```python
from build123d import *

# Parameters (mm, degrees)
BOSS_EXTRUDE1_DEPTH = 2
BOSS_EXTRUDE2_START = 10
SKETCH3_R           = 5
SKETCH3_R_2         = 3
BOSS_EXTRUDE2_DEPTH = 10
SKETCH4_R           = 5
SKETCH4_R_2         = 3
BOSS_EXTRUDE3_DEPTH = 10


with BuildPart() as part:
    # Sketch2 → Boss-Extrude1 (new, symmetric)
    with BuildSketch(Plane.XY):
        with BuildLine():
            Line((-17.054545455, 5), (7.945454545, 5))
            ThreePointArc((7.945454545, 5), (12.945454545, 0), (7.945454545, -5))
            Line((7.945454545, -5), (-17.054545455, -5))
            ThreePointArc((-17.054545455, -5), (-22.054545455, 0), (-17.054545455, 5))
        make_face()
    extrude(amount=BOSS_EXTRUDE1_DEPTH, both=True)

    # Sketch3 → Boss-Extrude2 (add)
    with BuildSketch(Plane.XY.offset(2).offset(BOSS_EXTRUDE2_START)):
        with Locations(Location((-17.054545455, 0, 0), (0, 0, 270))):
            Circle(SKETCH3_R)
        with Locations((-17.054545455, 0)):
            Circle(SKETCH3_R_2, mode=Mode.SUBTRACT)
    extrude(amount=-BOSS_EXTRUDE2_DEPTH)

    # Sketch4 → Boss-Extrude3 (add)
    with BuildSketch(Plane(origin=(0, 0, -2), x_dir=(-1, 0, 0), z_dir=(0, 0, -1))):
        with Locations((-7.945454545, 0)):
            Circle(SKETCH4_R)
        with Locations((-7.945454545, 0)):
            Circle(SKETCH4_R_2, mode=Mode.SUBTRACT)
    extrude(amount=BOSS_EXTRUDE3_DEPTH)


solid = part.part
```
Can you work these out from the model? Positions are in its coordinate system, mm. A direction names the side the tool comes from. Coordinates: 2 decimals unless noted, no trailing zeros. Write each loop counter-clockwise with the first axis right and the second up, starting at its lowest first coordinate (ties: lowest second). Pieces come first, ordered by that corner, then holes. Notation, with made-up numbers: M -11.75,-6 L 7.25,-6 A23 ccw 7.25,14 Z; hole C 54,-37.75 d8. An arc over 180 degrees is marked long. Write item = value, one per line. Start each with the question number.
Q1. On a 3-axis mill with a long thin cutter (end or side, diameter ignored), from which of +Z, -Z, +X, -X, +Y, -Y can I reach the whole of each face in a straight line? I mean faces 4 (the face through (-14.283, -1.149, 7.07)), 5 (the face through (-5, 5, 0)), 6 (the face through (10.943, 0.132, -6.93)). Say none if no direction works.
Q2. If we section it at B-B, the plane z = 4.5: Write out the boundary of the cut face in (x, y).
Q3. If I drill on L1, parallel to Z at x = 11, y = 0.25; L2, parallel to Z at x = -14, y = -3.75; L3, parallel to Y at x = 10, z = -11, over which ranges is the centre line in solid material (lowest first)? Write a range as [from, to].
Q4. If we section it at A-A, the plane y = 0: Write out the boundary of the cut face in (x, z), then the cut area to 3 significant figures.
Q5. If we section it at C-C, the plane x = 3.5: Write out the boundary of the cut face in (y, z), then the cut area to 3 significant figures.
Q6. Thinking about a two-plate mould opening in X: for faces 1 (the face through (-20.3, 0.1, 12)), 2 (the face through (-17, 0, 2)), 3 (the face through (12.94, 0.22, -6.46)), which applies, released by +X, released by -X, zero draft, split by the parting line, or undercut?
Q7. If we section it at D-D, the plane z = 0: Write out the boundary of the cut face in (x, y).
Q8. I'm going to push flat-ended pins straight in: pin 1 (1 mm diameter, centred on x = -3.5, y = 2.5, fed in from +Z); pin 2 (5 mm diameter, centred on y = -0.5, z = -6, fed in from -X); pin 3 (2 mm diameter, centred on y = 3, z = 7.5, fed in from -X). Where does each tip first touch, or does it pass through?
Check sheet entries:
q1.face_4 = +Z
q1.face_5 = +Z, -Z, +X, -X, +Y
q1.face_6 = -Z
q2.outline = C -17.05,0 d10; hole C -17.05,0 d6
q3.L1 = [-12, 2]
q3.L2 = [-2, 12]
q3.L3 = [-4.56, -2.19], [2.19, 4.56]
q4.outline = M -22.05,-2 L 2.95,-2 L 2.95,-12 L 4.95,-12 L 4.95,-2 L 10.95,-2 L 10.95,-12 L 12.95,-12 L 12.95,2 L -12.05,2 L -12.05,12 L -14.05,12 L -14.05,2 L -20.05,2 L -20.05,12 L -22.05,12 Z
q4.area = 220 mm²
q5.outline = M -5,-2 L -2.29,-2 L -2.29,-12 L 2.29,-12 L 2.29,-2 L 5,-2 L 5,2 L -5,2 Z
q5.area = 85.8 mm²
q6.face_1 = zero draft
q6.face_2 = undercut
q6.face_3 = split by the parting line
q7.outline = M -17.05,-5 L 7.95,-5 A5 ccw 7.95,5 L -17.05,5 A5 ccw Z
q8.pin_1 = 2
q8.pin_2 = 2.95
q8.pin_3 = -21.64
